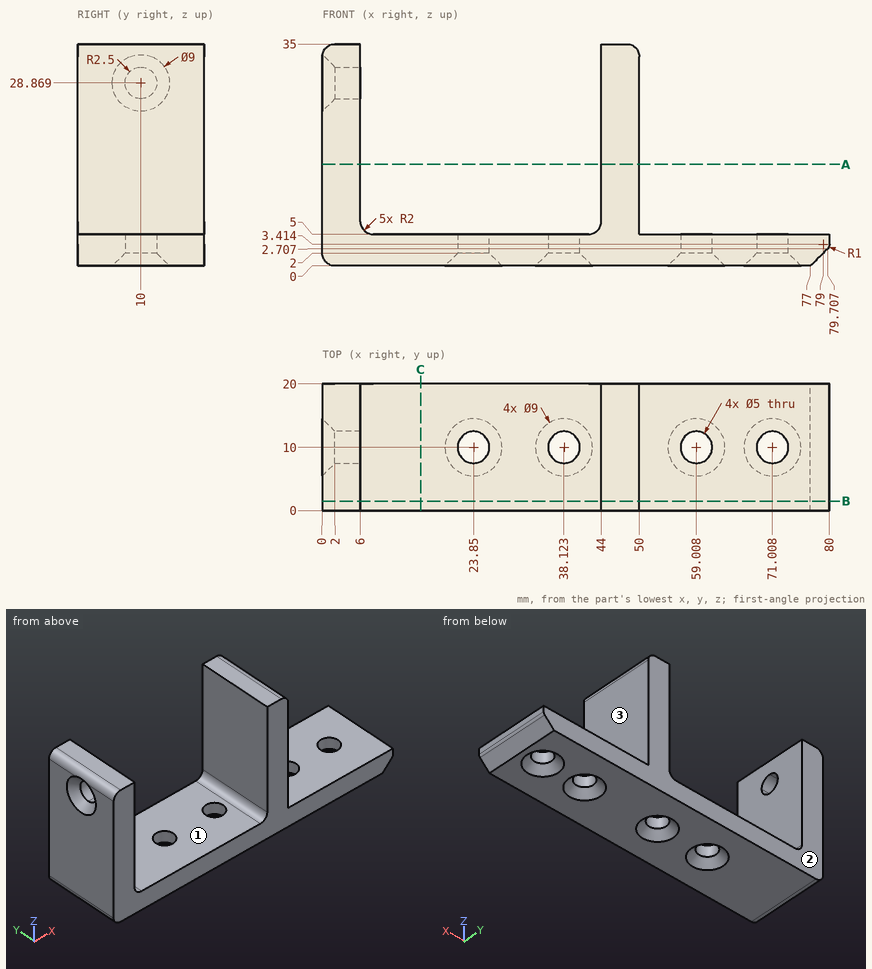
For this review, use the dimensioned drawing (mm, ordinates from the lowest corner) and the shaded views. A direction names the side the tool comes from. Give positions to 0.01 mm unless a question says otherwise; leave off trailing zeros. Order: outer loops, then holes, each group sorted by start corner. A loop starts at its lowest first (then second) coordinate and runs counter-clockwise, first axis right, second up. Notation, with made-up numbers: M 2.25,82 L 27.25,82 A33 ccw 27.25,119 Z; hole C 84.5,-34 d6. An arc over 180 degrees is marked long. Use one line per item in the form item = value. Start each with the question number.
Item 1: To check wall thickness, follow line 1 along X through (y, z) = (19.25, 22); line 2 along Z through (x, y) = (38, 16.5); line 3 along Y through (x, z) = (70, 3.5). State the ranges of each line that lie inside material, in increasing order. Write a range as from..to.
Item 2: We need section B-B on y = 1.5. Give the boundary of the cut face in (x, z) (1 decimal).
Item 3: We need section C-C on x = 15.5. Give the boundary of the cut face in (y, z), plus the area to 3 significant figures.
Item 4: Insertion check: pin 1 Ø3 at (x, y) = (23.85, 10) entering from -Z; pin 2 Ø6 at (x, y) = (71.01, 10) entering from +Z; pin 3 Ø6 at (y, z) = (6, 16.5) entering from +X; pin 4 Ø1.5 at (x, y) = (36, 10) entering from -Z (1 decimal). Each pin has a flat end and moves straight along its axis. Give the tip position at first contact, or say it passes through.
Item 5: We need section A-A on z = 16. Give the boundary of the cut face in (x, y).
Item 6: For the marked faces 1, 2 and 3, list the 3-axis set-ups (+Z, -Z, +X, -X, +Y, -Y) from which the entire face can be reached by the end or side of a thin tool; tool diameter is ignored.
Completed:
q1.line_1 = 0..6, 44..50
q1.line_2 = 0..5
q1.line_3 = 0..7.71, 12.29..20
q2.outline = M 0,2 A2 ccw 2,0 L 77,0 L 79.7,2.7 A1 ccw 80,3.4 L 80,5 L 50,5 L 50,33 A2 ccw 48,35 L 44,35 L 44,7 A2 cw 42,5 L 8,5 A2 cw 6,7 L 6,35 L 2,35 A2 ccw 0,33 Z
q3.outline = M 0,0 L 20,0 L 20,5 L 0,5 Z
q3.area = 100 mm²
q4.pin_1 = through
q4.pin_2 = 5
q4.pin_3 = 50
q4.pin_4 = 1.6
q5.outline = M 0,0 L 6,0 L 6,20 L 0,20 Z; M 44,0 L 50,0 L 50,20 L 44,20 Z
q6.face_1 = +Z, +Y, -Y
q6.face_2 = +Z, -Z, +X, -X, +Y
q6.face_3 = +Z, +X, +Y, -Y
